from build123d import *

# Parameters (mm, degrees)
EXTRU_MINCE1_DEPTH      = 37.5
ESQUISSE2_R             = 1.5
ENL_V_MAT_EXTRU_1_DEPTH = 3


with BuildPart() as part:
    # Esquisse1 → Extru.-Mince1 (new, symmetric)
    with BuildSketch(Plane.XY):
        Polygon((-17.75, 19.5), (-17.75, 0), (17.75, 0), (17.75, 19.5), (16.25, 19.5), (16.25, 1.5), (-16.25, 1.5), (-16.25, 19.5), align=None)
    extrude(amount=EXTRU_MINCE1_DEPTH, both=True)

    # Esquisse2 → Enlèv. mat.-Extru.1 (cut)
    with BuildSketch(Plane.XZ):
        with Locations(Location((-2.75, 15, 0), (0, 0, 270))):
            Circle(ESQUISSE2_R)
        with Locations(Location((-2.75, -15, 0), (0, 0, 90))):
            Circle(ESQUISSE2_R)
        with BuildLine():
            Line((11.75, 20), (17.75, 20))
            Line((17.75, 20), (17.75, -4))
            Line((17.75, -4), (11.75, -4))
            ThreePointArc((11.75, -4), (8.921572875, -2.828427125), (7.75, 0))
            Line((7.75, 0), (7.75, 16))
            ThreePointArc((7.75, 16), (8.921572875, 18.828427125), (11.75, 20))
        make_face()
    extrude(amount=-ENL_V_MAT_EXTRU_1_DEPTH, mode=Mode.SUBTRACT)


solid = part.part
CAD build for the part. Positions are in the model's coordinates, mm. A direction names the side the tool comes from. Round coordinates to 2 decimals unless told otherwise and drop trailing zeros. Order: outer loops, then holes, each group sorted by start corner. A loop starts at its lowest first (then second) coordinate and runs counter-clockwise, first axis right, second up. Notation, with made-up numbers: (18, -2) -> (49, -2) arc R22 cw to (49, 11) -> close; hole circle Ø2 at (-8.5, -32.5). An arc over 180 degrees is marked (long way). Write each question's results on one line, items separated by ' | '.
1. Cut at C-C (x = -3.5). Give the cut face in (y, z), plus the area to 3 significant figures.
Findings below:
outline: (0, -37.5) -> (1.5, -37.5) -> (1.5, -16.3) -> (0, -16.3) -> close; (0, -13.7) -> (1.5, -13.7) -> (1.5, 13.7) -> (0, 13.7) -> close; (0, 16.3) -> (1.5, 16.3) -> (1.5, 37.5) -> (0, 37.5) -> close | area: 105 mm²
2. Cut at A-A (z = 2.5). Give the cut face in (x, y).
Findings below:
outline: (-17.75, 0) -> (7.75, 0) -> (7.75, 1.5) -> (-16.25, 1.5) -> (-16.25, 19.5) -> (-17.75, 19.5) -> close; (16.25, 3) -> (17.75, 3) -> (17.75, 19.5) -> (16.25, 19.5) -> close
3. Flat gauge pins, fed straight in: P1, Ø4, axis at x = -3, z = 16.5, coming from the +Y side; P2, Ø1.2, axis at y = 0.5, z = 7.5, coming from the +X side; P3, Ø0.8, axis at x = 17, z = 7, coming from the -Y side. Where does each tip first touch, or does it go through?
Findings below:
P1: stops at y = 1.5 | P2: stops at x = 7.75 | P3: stops at y = 3
4. Cut at D-D (z = 15). Give the cut face in (x, y), plus the area to 3 significant figures.
Findings below:
outline: (-17.75, 0) -> (-4.25, 0) -> (-4.25, 1.5) -> (-16.25, 1.5) -> (-16.25, 19.5) -> (-17.75, 19.5) -> close; (-1.25, 0) -> (7.75, 0) -> (7.75, 1.5) -> (-1.25, 1.5) -> close; (16.25, 3) -> (17.75, 3) -> (17.75, 19.5) -> (16.25, 19.5) -> close | area: 85.5 mm²
5. Wall check: line 1 along X through (y, z) = (5.25, 26.5); line 2 along X through (y, z) = (0.55, 15); line 3 along Y through (x, z) = (-1.5, 10.5). Give the ranges that are in metal, low to high. Write a range as [from, to].
Findings below:
line 1: x = [-17.75, -16.25], [16.25, 17.75] | line 2: x = [-17.75, -4.25], [-1.25, 7.75] | line 3: y = [0, 1.5]
6. 3-axis set-ups, long thin cutter, end or side, ignore diameter. For faces 1 (the face through (7.75, 1, 8)), 2 (the face through (0, 1.5, 1)), 3 (the face through (15, 1, 20)): which of +Z, -Z, +X, -X, +Y, -Y reach the whole face in a straight line?
Findings below:
face 1: +X, +Y, -Y | face 2: +Z, -Z, +Y | face 3: +X, -Y
7. Cut at B-B (y = 12). Give the cut face in (x, z), plus the area to 3 significant figures.
Findings below:
outline: (-17.75, -37.5) -> (-16.25, -37.5) -> (-16.25, 37.5) -> (-17.75, 37.5) -> close; (16.25, -37.5) -> (17.75, -37.5) -> (17.75, 37.5) -> (16.25, 37.5) -> close | area: 225 mm²
8. Pull direction Z, two halves, no side cores. Call faces 4 (the face through (8.953, 0.74, -2.859)), 5 (the face through (-16.25, 10, 1)), 6 (the face through (0, 1, 37.5)): pulls with the +Z half, pulls with the -Z half, needs draft (parallel to the pull), parting line crosses it, or undercut.
Findings below:
face 4: undercut | face 5: needs draft | face 6: pulls with the +Z half
